Work out the finished part from the listing and answer in its coordinate system (mm). Face numbers are marked on the shaded views. A direction names the side the tool comes from. Round coordinates to 2 decimals unless told otherwise and drop trailing zeros. Order: outer loops, then holes, each group sorted by start corner. A loop starts at its lowest first (then second) coordinate and runs counter-clockwise, first axis right, second up. Notation, with made-up numbers: (0.25, -9.75) -> (55.25, -9.75) arc R16 cw to (55.25, 15.25) -> close; hole circle Ø8 at (80.25, 44). An arc over 180 degrees is marked (long way). Use a Markdown table: item, result. Add a question column.
Item 1: A cutting plane is placed at C-C, the plane y = -1.95. Determine the outline of the cut face in (x, z).
Item 2: A cutting plane is placed at D-D, the plane y = 1. Determine the outline of the cut face in (x, z), plus the area to 3 significant figures.
Item 3: A cutting plane is placed at B-B, the plane x = 26.5. Determine the outline of the cut face in (y, z).
Item 4: A tool of negligible diameter and unlimited length cuts with its end or side. For the marked faces 1 and 2, from which of +Z, -Z, +X, -X, +Y, -Y can it reach the whole face along a straight path? Write none if from no direction.
Item 5: Flat-ended cylindrical pins translate along their axes: P1, Ø2, axis at y = -0.5, z = -33, coming from the -X side; P2, Ø6.5, axis at x = 15, z = -2.5, coming from the -Y side. Find the tip coordinate at first contact, or state that the pin passes through.
Item 6: A cutting plane is placed at A-A, the plane z = -48.25. Determine the outline of the cut face in (x, y), plus the area to 3 significant figures.
Item 7: Find the intervals of material crossed by L1, parallel to Z at x = 16.5, y = 1; L2, parallel to Y at x = 28.25, z = -45; L3, parallel to Z at x = 21.5, y = 0.5, in increasing order. Write a range as [from, to].
from build123d import *

# Parameters (mm, degrees)
SKETCH1_W           = 28
SKETCH1_H           = 26.15
BOSS_EXTRUDE1_DEPTH = 2
SKETCH12_W          = 52.3
SKETCH12_H          = 7
BOSS_EXTRUDE2_DEPTH = 2
SKETCH13_W          = 30
SKETCH13_H          = 36.1
CUT_EXTRUDE3_DEPTH  = 2
SKETCH15_W          = 2
SKETCH15_H          = 36.1
BOSS_EXTRUDE3_DEPTH = 2


with BuildPart() as part:
    # Sketch1 → Boss-Extrude1 (new body)
    # profile 1 of 2: a face of its own
    with BuildSketch(Plane(origin=(0, 0, 0), x_dir=(1, 0, 0), z_dir=(0, 1, 0))):
        with Locations((14, 39.225)):
            Rectangle(SKETCH1_W, SKETCH1_H)
        with BuildLine():
            Line((19.05, 46.2), (4.05, 46.2))
            ThreePointArc((4.05, 46.2), (2, 48.25), (4.05, 50.3))
            Line((4.05, 50.3), (19.05, 50.3))
            ThreePointArc((19.05, 50.3), (21.1, 48.25), (19.05, 46.2))
        make_face(mode=Mode.SUBTRACT)
    # profile 2 of 2: a face of its own
    with BuildSketch(Plane(origin=(0, 0, 0), x_dir=(1, 0, 0), z_dir=(0, 1, 0))):
        with Locations((14, 13.075)):
            Rectangle(SKETCH1_W, SKETCH1_H)
        with BuildLine():
            ThreePointArc((4.05, 2), (2, 4.05), (4.05, 6.1))
            Line((4.05, 6.1), (19.05, 6.1))
            ThreePointArc((19.05, 6.1), (21.1, 4.05), (19.05, 2))
            Line((19.05, 2), (4.05, 2))
        make_face(mode=Mode.SUBTRACT)
    extrude(amount=BOSS_EXTRUDE1_DEPTH)

    # Sketch12 → Boss-Extrude2 (add)
    with BuildSketch(Plane(origin=(28, 0, 0), x_dir=(0, 0, -1), z_dir=(1, 0, 0))):
        with Locations((26.15, -1.5)):
            Rectangle(SKETCH12_W, SKETCH12_H)
        with BuildLine():
            Line((6.15, -0.9), (46.15, -0.9))
            ThreePointArc((46.15, -0.9), (47.2, -1.95), (46.15, -3))
            Line((46.15, -3), (6.15, -3))
            ThreePointArc((6.15, -3), (5.1, -1.95), (6.15, -0.9))
        make_face(mode=Mode.SUBTRACT)
    extrude(amount=BOSS_EXTRUDE2_DEPTH)

    # Sketch13 → Cut-Extrude3 (cut)
    with BuildSketch(Plane(origin=(0, 2, 0), x_dir=(1, 0, 0), z_dir=(0, 1, 0))):
        with Locations((15, 26.15)):
            Rectangle(SKETCH13_W, SKETCH13_H)
    extrude(amount=-CUT_EXTRUDE3_DEPTH, mode=Mode.SUBTRACT)

    # Sketch15 → Boss-Extrude3 (add)
    with BuildSketch(Plane(origin=(0, 0, 0), x_dir=(1, 0, 0), z_dir=(0, 1, 0))):
        with Locations((29, 26.15)):
            Rectangle(SKETCH15_W, SKETCH15_H)
    extrude(amount=BOSS_EXTRUDE3_DEPTH)


solid = part.part
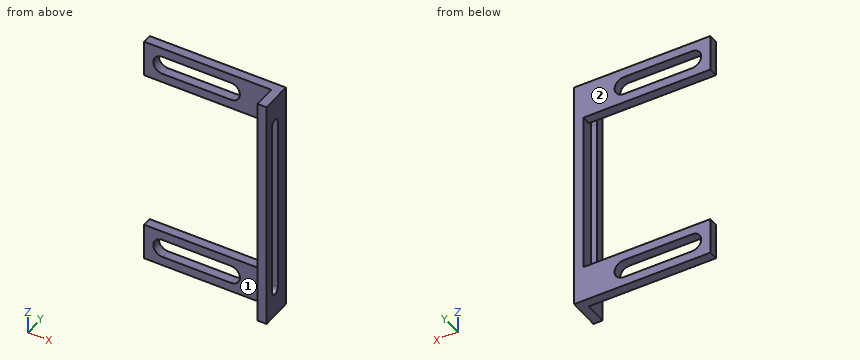
Reported:
| question | item | result |
|---|---|---|
| 1 | outline | (28, -52.3) -> (30, -52.3) -> (30, -47.2) -> (28, -47.2) -> close; (28, -5.1) -> (30, -5.1) -> (30, 0) -> (28, 0) -> close |
| 2 | outline | (0, -52.3) -> (30, -52.3) -> (30, 0) -> (0, 0) -> (0, -8.1) -> (28, -8.1) -> (28, -44.2) -> (0, -44.2) -> close; hole (4.05, -50.3) -> (19.05, -50.3) arc R2.05 ccw to (19.05, -46.2) -> (4.05, -46.2) arc R2.05 ccw to start; hole (4.05, -6.1) -> (19.05, -6.1) arc R2.05 ccw to (19.05, -2) -> (4.05, -2) arc R2.05 ccw to start |
| 2 | area | 409 mm² |
| 3 | outline | (0, -52.3) -> (2, -52.3) -> (2, -44.2) -> (0, -44.2) -> close; (0, -8.1) -> (2, -8.1) -> (2, 0) -> (0, 0) -> close |
| 4 | face 1 | +Z, -Z, -X, -Y |
| 4 | face 2 | +Z, -Z, +X, -X, +Y |
| 5 | P1 | x = 28 |
| 5 | P2 | y = 0 |
| 6 | outline | (0, 0) -> (2, 0) -> (2, 2) -> (0, 2) -> close; (21.1, 0) -> (28, 0) -> (28, -5) -> (30, -5) -> (30, 2) -> (21.1, 2) -> close |
| 6 | area | 31.8 mm² |
| 7 | L1 | [-52.3, -50.3], [-46.2, -44.2], [-8.1, -6.1], [-2, 0] |
| 7 | L2 | [-5, -3], [-0.9, 2] |
| 7 | L3 | [-52.3, -44.2], [-8.1, 0] |
